Could you check a few things on this model? Use its own coordinates, in mm. A direction names the side the tool comes from. Give positions to 0.01 mm unless a question says otherwise; leave off trailing zeros. Order: outer loops, then holes, each group sorted by start corner. A loop starts at its lowest first (then second) coordinate and runs counter-clockwise, first axis right, second up.
(1) Imagine slicing it at A-A, the plane x = 10.5. Write out the boundary of the cut face in (y, z) (3 decimals), then the cut area to 3 significant figures.
(2) If I drill on probe 1 along Y at (x, z) = (24.5, 681.5) (3 decimals); probe 2 along Y at (x, z) = (20.5, 851) (3 decimals), over which ranges is the centre line in solid material (lowest first)?
(3) Imagine slicing it at D-D, the plane z = 151. Write out the boundary of the cut face in (x, y) (3 decimals).
(4) Will these pins go through, and if not, where does the flat tip stop? pin 1 (1 mm diameter, centred on x = 17.5, y = 74.5, fed in from -Z) (3 decimals); pin 2 (3.5 mm diameter, centred on x = 12.5, y = 75.5, fed in from +Z) (3 decimals); pin 3 (5 mm diameter, centred on y = 37.5, z = 623, fed in from -X); pin 4 (4 mm diameter, centred on x = 3, y = 46, fed in from -Z).
(5) On a 3-axis mill with a long thin cutter (end or side, diameter ignored), from which of +Z, -Z, +X, -X, +Y, -Y can I reach the whole of each face in a straight line? I mean faces 4 (the flat face through (14, 73.025, 466)), 5 (the flat face through (13, 0, 463)). Say none if no direction works.
(6) If we mould it in two halves opening along Y, with no side actions, what happens to faces 1 (the flat face through (0, 39, 463)), 2 (the flat face through (13, 76.2, 463)), 3 (the flat face through (14, 3.175, 463))? For each: released by +Y, released by -Y, zero draft, split by the parting line, or undercut.
(7) Imagine slicing it at C-C, the plane y = 51.5. Write out the boundary of the cut face in (x, z) (3 decimals).
(8) Imagine slicing it at B-B, the plane z = 589. Write out the boundary of the cut face in (x, y) (3 decimals).
Autodesk Inventor part; units mm, degrees
ref_plane "YZ Plane" through (0, 0, 0) normal (1, 0, 0) x (0, 1, 0)
ref_plane "XZ Plane" through (0, 0, 0) normal (0, 1, 0) x (-1, 0, 0)
ref_plane "XY Plane" through (0, 0, 0) normal (0, 0, 1) x (1, 0, 0)
sketch "Sketch1" plane through (0, 0, 0) normal (0, 0, 1) x (1, 0, 0)
  line L0 (0, 0) -> (25.4, 0)
  line L1 (25.4, 76.2) -> (0, 76.2)
  line L2 (0, 76.2) -> (0, 0)
  line L3 (25.4, 3.175) -> (3.175, 3.175)
  line L4 (3.175, 3.175) -> (3.175, 73.025)
  line L5 (3.175, 73.025) -> (25.4, 73.025)
  line L6 (25.4, 0) -> (25.4, 3.175)
  line L7 (25.4, 73.025) -> (25.4, 76.2)
  dimension "d0" = 76.2
  dimension "d1" = 25.4
  dimension "d2" = 3.175
  dimension "d3" = 3.175
  dimension "d4" = 3.175
extrude "Extrusion1" add sketch "Sketch1" along normal blind 939.8
sketch "Sketch2" plane through (0, 76.2, 0) normal (0, 1, 0) x (1, 0, 0)
  line L0 (0, -939.8) -> (25.4, -939.8)
  line L1 (25.4, 0) -> (25.4, -939.8)
  line L2 (25.4, 0) -> (0, 0)
  line L3 (0, 0) -> (0, -939.8)
  line L4 (0, -939.8) -> (25.4, -914.4)
  line L5 (0, 0) -> (25.4, -25.4)
  line L6 (3.175, -936.625) -> (3.175, -771.525)
  line L7 (3.175, -771.525) -> (25.4, -771.525)
  line L8 (3.175, -3.175) -> (3.175, -168.275)
  line L9 (3.175, -168.275) -> (25.4, -168.275)
  dimension "d7" = 45
  dimension "d8" = 3.175
  dimension "d9" = 165.1
  dimension "d10" = 165.1
extrude "Extrusion2" cut sketch "Sketch2" against normal through all contours L4 L1 L0 | L2 L1 L5
extrude "Extrusion3" cut sketch "Sketch2" against normal up to next contours L6 L7 L1 L4 | L5 L1 L9 L8
equation "\"d3\" = d2"
equation "\"d4\" = d2"
equation "\"d10\" = d9"
properties part number "frame U 1 by 3 long"
Answer block:
1. outline: (0, 10.5) - (3.175, 10.5) - (3.175, 929.3) - (0, 929.3) - close; (73.025, 168.275) - (76.2, 168.275) - (76.2, 771.525) - (73.025, 771.525) - close
1. area: 4,830 mm2
2. probe 1: y = 0 to 3.175, 73.025 to 76.2
2. probe 2: y = 0 to 3.175
3. outline: (0, 0) - (25.4, 0) - (25.4, 3.175) - (3.175, 3.175) - (3.175, 76.2) - (0, 76.2) - close
4. pin 1: stops at z = 168.275
4. pin 2: stops at z = 771.525
4. pin 3: stops at x = 0
4. pin 4: stops at z = 1
5. face 4: +Z, -Z, +X
5. face 5: +Z, -Z, +X, -X, -Y
6. face 1: zero draft
6. face 2: released by +Y
6. face 3: undercut
7. outline: (0, 0) - (3.175, 3.175) - (3.175, 936.625) - (0, 939.8) - close
8. outline: (0, 0) - (25.4, 0) - (25.4, 3.175) - (3.175, 3.175) - (3.175, 73.025) - (25.4, 73.025) - (25.4, 76.2) - (0, 76.2) - close
